Can you work these out from the model? Positions are in its coordinate system, mm. A direction names the side the tool comes from. Give positions to 0.01 mm unless a question says otherwise; leave off trailing zeros. Loops run counter-clockwise (first coordinate to the right, second up) from the corner with the lowest first, then second, coordinate; pieces in that order, holes last. Notation, with made-up numbers: (59, 48.5) - (66, 48.5) arc R15 cw to (66, 66.5) - close; hole circle Ø8 at (4, -23). An arc over 180 degrees is marked (long way). Answer as a JSON object with one key per item and string values.
```python
from build123d import *

# Parameters (mm, degrees)
F1_DEPTH  = 2.5
F2_R      = 1.5
F3_DEPTH  = 2.501
F4_W      = 20
F4_H      = 2.5
F5_DEPTH  = 5
F7_W      = 80
F7_H      = 20
F8_DEPTH  = 2.5
F9_W      = 22.5
F9_H      = 20
F10_DEPTH = 2.5


with BuildPart() as f1:
    # F0 (on Top) → F1 (new body)
    with BuildSketch(Plane.XY):
        Polygon((35, -3), (35, 3), (-35, 3), (-35, -3), (-35, -23), (35, -23), align=None)
    extrude(amount=F1_DEPTH)

    # F2 (on face) → F3 (cut, through all)
    with BuildSketch(Plane(origin=(0, 0, 0), x_dir=(1, 0, 0), z_dir=(0, 0, -1))):
        with Locations((-25, 0)):
            Circle(F2_R)
        with Locations((25, 0)):
            Circle(F2_R)
    extrude(amount=-F3_DEPTH, mode=Mode.SUBTRACT)

    # F4 (on face) → F5 (join)
    with BuildSketch(Plane(origin=(-35, 0, 0), x_dir=(0, -1, 0), z_dir=(-1, 0, 0))):
        with Locations((13, 1.25)):
            Rectangle(F4_W, F4_H)
    extrude(amount=F5_DEPTH)

    # F6: F1 across plane


with BuildPart() as f1_1:
    add(f1.part)
    add(f1.part.mirror(Plane.YZ))

    # F7 (on face) → F8 (join)
    with BuildSketch(Plane.XZ.offset(23)):
        with Locations((0, 10)):
            Rectangle(F7_W, F7_H)
    extrude(amount=F8_DEPTH)

    # F9 (on face) → F10 (join)
    with BuildSketch(Plane.YZ.offset(40)):
        with Locations((-14.25, 10)):
            Rectangle(F9_W, F9_H)
    extrude(amount=F10_DEPTH)

    # F11: F1 across plane


with BuildPart() as f1_2:
    add(f1_1.part)
    add(f1_1.part.mirror(Plane.YZ))


solid = f1_2.part
```
1) I need wall thicknesses on L1, parallel to Y at x = 25, z = 1.4; L2, parallel to X at y = -6.5, z = 17.5; L3, parallel to Y at x = 5, z = 5.75. Which ranges of each line are inside material? Lowest first, please.
Check sheet entries:
{"L1": "-25.5 to -1.5, 1.5 to 3", "L2": "-42.5 to -40, 40 to 42.5", "L3": "-25.5 to -23"}
2) Imagine slicing it at B-B on z = 6.25. Write out the boundary of the cut face in (x, y).
Check sheet entries:
{"outline": "(-42.5, -25.5) - (42.5, -25.5) - (42.5, -3) - (40, -3) - (40, -23) - (-40, -23) - (-40, -3) - (-42.5, -3) - close"}
3) Imagine slicing it at A-A on y = 0. Write out the boundary of the cut face in (x, z), and give its area (3 significant figures).
Check sheet entries:
{"outline": "(-35, 0) - (-26.5, 0) - (-26.5, 2.5) - (-35, 2.5) - close; (-23.5, 0) - (23.5, 0) - (23.5, 2.5) - (-23.5, 2.5) - close; (26.5, 0) - (35, 0) - (35, 2.5) - (26.5, 2.5) - close", "area": "160 mm2"}
4) If we mould it in two halves opening along Y, with no side actions, what happens to faces 4 (the cylindrical face through (23.5, -0.07, 1.23)), 5 (the flat face through (40.4, -3, 7.6)), 6 (the cylindrical face through (-26.5, -0.07, 1.23)), 7 (the flat face through (-1, -10, 2.5))? For each: released by +Y, released by -Y, zero draft, split by the parting line, or undercut.
Check sheet entries:
{"face 4": "undercut", "face 5": "released by +Y", "face 6": "undercut", "face 7": "zero draft"}
5) Imagine slicing it at C-C on x = -25. Write out the boundary of the cut face in (y, z), and give its area (4 significant figures).
Check sheet entries:
{"outline": "(-25.5, 0) - (-1.5, 0) - (-1.5, 2.5) - (-23, 2.5) - (-23, 20) - (-25.5, 20) - close; (1.5, 0) - (3, 0) - (3, 2.5) - (1.5, 2.5) - close", "area": "107.5 mm2"}
6) I'm going to push flat-ended pins straight in: P1, Ø2, axis at y = 1.5, z = 1.5, coming from the +X side; P2, Ø4, axis at x = 39, z = 9, coming from the +Y side; P3, Ø6, axis at x = -20, z = 11.5, coming from the +Y side; P4, Ø1.8, axis at x = 25, y = 0, coming from the -Z side. Where does each tip first touch, or does it pass through?
Check sheet entries:
{"P1": "x = 35", "P2": "y = -3", "P3": "y = -23", "P4": "through"}
7) Imagine slicing it at D-D on y = -19. Write out the boundary of the cut face in (x, z), and give its area (3 significant figures).
Check sheet entries:
{"outline": "(-42.5, 0) - (42.5, 0) - (42.5, 20) - (40, 20) - (40, 2.5) - (-40, 2.5) - (-40, 20) - (-42.5, 20) - close", "area": "300 mm2"}
8) Which directions (+Z, -Z, +X, -X, +Y, -Y) give clear straight access to the entire face, cutting with the end or side of a thin tool? Please do faces 1 (the flat face through (-40.4, -3, 7.6)), 2 (the flat face through (35, 0, 1)), 3 (the flat face through (40, -13, 11)).
Check sheet entries:
{"face 1": "+Z, -Z, -X, +Y", "face 2": "+Z, -Z, +X, +Y", "face 3": "+Z, +Y"}
